For this review, use the dimensioned drawing (mm, ordinates from the lowest corner) and the shaded views. A direction names the side the tool comes from. Round coordinates to 2 decimals unless told otherwise and drop trailing zeros. Order: outer loops, then holes, each group sorted by start corner. A loop starts at its lowest first (then second) coordinate and runs counter-clockwise, first axis right, second up. Notation, with made-up numbers: (10.5, -16) -> (54.5, -16) arc R22 cw to (54.5, -7) -> close; hole circle Ø11 at (-0.5, 75.25). An arc over 180 degrees is marked (long way). Use a Markdown table: item, result. Add a question column.
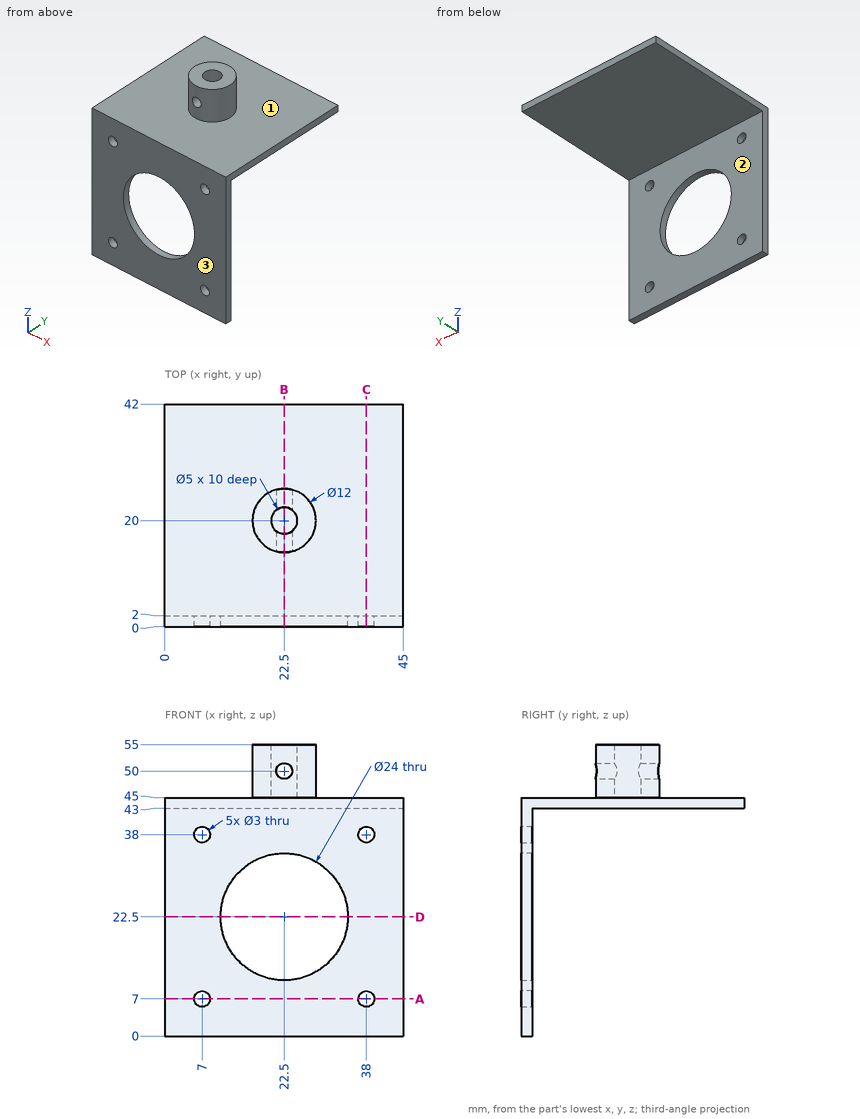
Q1. Add section A-A (z = 7). Write out the cut boundary in (x, y), then the cut area to 3 significant figures.
Q2. Add section C-C (x = 38). Write out the cut boundary in (y, z), then the cut area to 3 significant figures.
Q3. Wall thickness on line 1 (X direction, y = 1, z = 38); line 2 (Z direction, x = 11, y = 40): over which ranges is each line inside the solid? List them lowest first. Write a range as [from, to].
Q4. Add section B-B (x = 22.5). Write out the cut boundary in (y, z).
Q5. Insertion check: pin 1 (1.5 mm diameter, centred on x = 39.5, z = 47, fed in from +Y); pin 2 (5 mm diameter, centred on x = 36, y = 7, fed in from -Z); pin 3 (5 mm diameter, centred on x = 38, z = 38, fed in from +Y). Each pin has a flat end and moves straight along its axis. Give the tip position at first contact, or say it passes through.
Q6. Add section D-D (z = 22.5). Write out the cut boundary in (x, y), then the cut area to 3 significant figures.
Q7. Machinability: for the marked faces 1, 2 and 3, which of the approach directions +Z, -Z, +X, -X, +Y, -Y give a long, thin tool a straight path to every point of the face, cutting with its end or side? Answer none if there is none.
Report:
| question | item | result |
|---|---|---|
| 1 | outline | (0, 0) -> (5.5, 0) -> (5.5, 2) -> (0, 2) -> close; (8.5, 0) -> (36.5, 0) -> (36.5, 2) -> (8.5, 2) -> close; (39.5, 0) -> (45, 0) -> (45, 2) -> (39.5, 2) -> close |
| 1 | area | 78.0 mm² |
| 2 | outline | (0, 0) -> (2, 0) -> (2, 5.5) -> (0, 5.5) -> close; (0, 8.5) -> (2, 8.5) -> (2, 36.5) -> (0, 36.5) -> close; (0, 39.5) -> (2, 39.5) -> (2, 43) -> (42, 43) -> (42, 45) -> (0, 45) -> close |
| 2 | area | 158 mm² |
| 3 | line 1 | x = [0, 5.5], [8.5, 36.5], [39.5, 45] |
| 3 | line 2 | z = [43, 45] |
| 4 | outline | (0, 0) -> (2, 0) -> (2, 10.5) -> (0, 10.5) -> close; (0, 34.5) -> (2, 34.5) -> (2, 43) -> (42, 43) -> (42, 45) -> (26, 45) -> (26, 48.5) -> (22.5, 48.5) -> (22.5, 45) -> (17.5, 45) -> (17.5, 48.5) -> (14, 48.5) -> (14, 45) -> (0, 45) -> close; (14, 51.5) -> (17.5, 51.5) -> (17.5, 55) -> (14, 55) -> close; (22.5, 51.5) -> (26, 51.5) -> (26, 55) -> (22.5, 55) -> close |
| 5 | pin 1 | passes through |
| 5 | pin 2 | stops at z = 43 |
| 5 | pin 3 | stops at y = 2 |
| 6 | outline | (0, 0) -> (10.5, 0) -> (10.5, 2) -> (0, 2) -> close; (34.5, 0) -> (45, 0) -> (45, 2) -> (34.5, 2) -> close |
| 6 | area | 42.0 mm² |
| 7 | face 1 | +Z |
| 7 | face 2 | -Z, +X, -X, +Y |
| 7 | face 3 | +Z, -Z, +X, -X, -Y |
